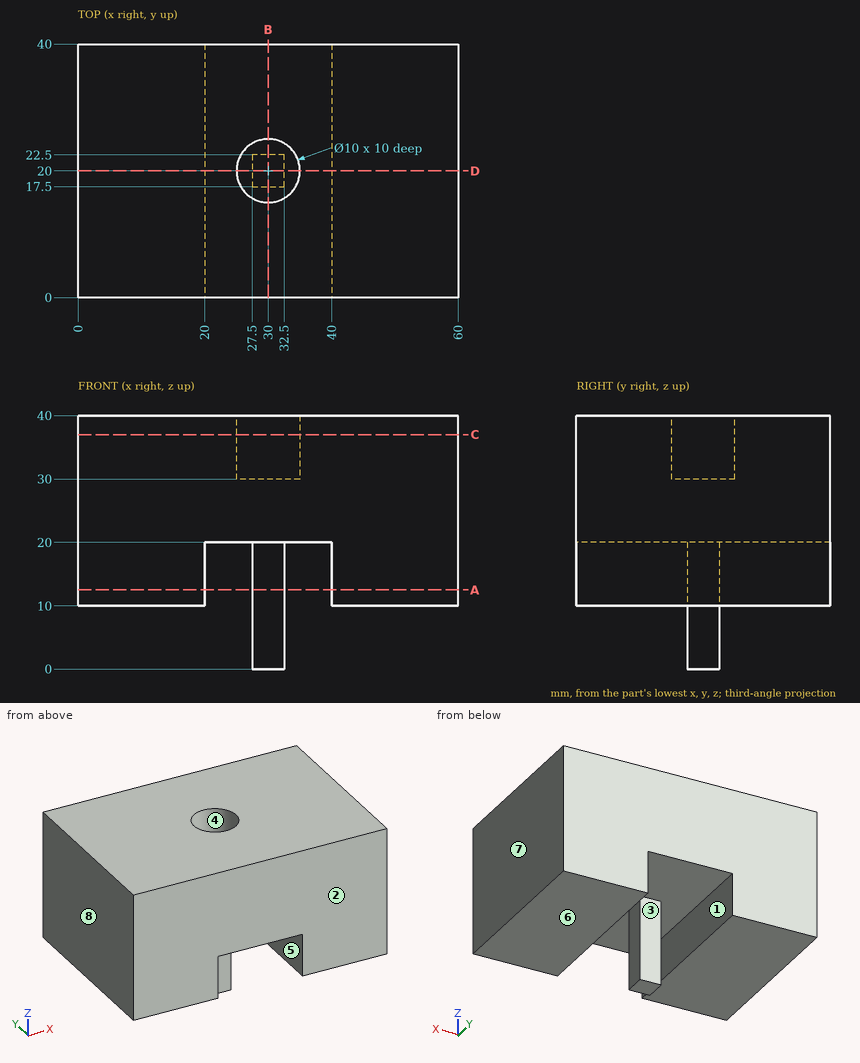
Source: three-view drawing plus pictorial views. Frame: mm from the lowest corner of the part. A direction names the side the tool comes from. Round coordinates to 2 decimals unless told otherwise and drop trailing zeros. Loops run counter-clockwise (first coordinate to the right, second up) from the corner with the lowest first, then second, coordinate; pieces in that order, holes last.
1. Section query D-D on y = 20. Output: boundary loops of the cut face in (x, z), and give its area (3 significant figures).
2. Mould query, pull axis X, two halves, no side actions, for the marked faces 5, 6, 7 and 8. Classes: released by +X, released by -X, zero draft, split by the parting line, or undercut.
3. Access query for the marked faces 1, 2, 3 and 4. Directions: +Z, -Z, +X, -X, +Y, -Y. A direction counts if a zero-diameter tool reaches every point of the face in a straight line with its end or side. Return the directions, or none.
4. Contact query for flat-ended pins moving along their axis: pin 1 (6 mm diameter, centred on x = 46.5, y = 30, fed in from -Z); pin 2 (2.5 mm diameter, centred on x = 30.5, z = 10.5, fed in from +Y); pin 3 (1 mm diameter, centred on x = 26.5, y = 11, fed in from -Z). Output: stop coordinate, or through.
5. Section query C-C on z = 37. Output: boundary loops of the cut face in (x, y), and give its area (3 significant figures).
6. Ray query, L1, parallel to X at y = 21, z = 12.5; L2, parallel to Y at x = 30, z = 36; L3, parallel to X at y = 13.5, z = 14.5. Return the intervals inside material, ascending.
7. Section query A-A on z = 12.5. Output: boundary loops of the cut face in (x, y).
8. Section query B-B on x = 30. Output: boundary loops of the cut face in (y, z).
Answers below:
1. outline: (0, 10) - (20, 10) - (20, 20) - (27.5, 20) - (27.5, 0) - (32.5, 0) - (32.5, 20) - (40, 20) - (40, 10) - (60, 10) - (60, 40) - (35, 40) - (35, 30) - (25, 30) - (25, 40) - (0, 40) - close
1. area: 1,600 mm2
2. face 5: undercut
2. face 6: zero draft
2. face 7: released by +X
2. face 8: released by -X
3. face 1: -Z, +Y, -Y
3. face 2: +Z, -Z, +X, -X, -Y
3. face 3: -Z, +Y
3. face 4: +Z
4. pin 1: stops at z = 10
4. pin 2: stops at y = 22.5
4. pin 3: stops at z = 20
5. outline: (0, 0) - (60, 0) - (60, 40) - (0, 40) - close; hole circle Ø10 at (30, 20)
5. area: 2,320 mm2
6. L1: x = 0 to 20, 27.5 to 32.5, 40 to 60
6. L2: y = 0 to 15, 25 to 40
6. L3: x = 0 to 20, 40 to 60
7. outline: (0, 0) - (20, 0) - (20, 40) - (0, 40) - close; (27.5, 17.5) - (32.5, 17.5) - (32.5, 22.5) - (27.5, 22.5) - close; (40, 0) - (60, 0) - (60, 40) - (40, 40) - close
8. outline: (0, 20) - (17.5, 20) - (17.5, 0) - (22.5, 0) - (22.5, 20) - (40, 20) - (40, 40) - (25, 40) - (25, 30) - (15, 30) - (15, 40) - (0, 40) - close
